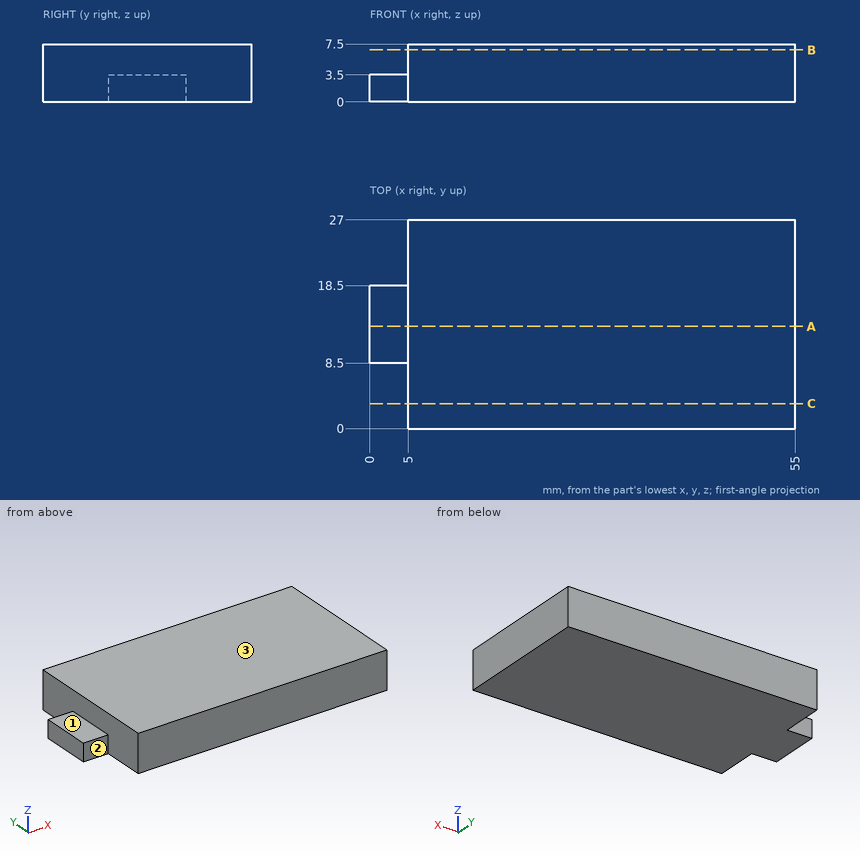
Here's the drawing with two shaded views (mm, measured from the low corner). I have some questions. A direction names the side the tool comes from. Coordinates: 2 decimals unless noted, no trailing zeros. Loops run counter-clockwise (first coordinate to the right, second up) from the corner with the lowest first, then second, coordinate; pieces in that order, holes last. Notation, with made-up numbers: (34, -6.5) -> (61, -6.5) arc R32 ccw to (61, 21.5) -> close; hole circle Ø3 at (-33.75, 30.25). An arc over 180 degrees is marked (long way). Put each result on its own line as item: value. Start each with the question number.
Q1. If I drill on line 1 (X direction, y = 12.25, z = 5.75), over which ranges is the centre line in solid material (lowest first)? Write a range as [from, to].
Q2. I want a section at C-C (y = 3.25). Write out the boundary of the cut face in (x, z).
Q3. I'm going to push flat-ended pins straight in: P1, Ø1.5, axis at x = 13.5, z = 5, coming from the -Y side; P2, Ø1.8, axis at x = 3, z = 2, coming from the +Y side; P3, Ø1.5, axis at y = 23.5, z = 5.5, coming from the -X side; P4, Ø1.5, axis at x = 3.5, y = 14.5, coming from the +Z side. Where does each tip first touch, or does it pass through?
Q4. I want a section at B-B (z = 6.75). Write out the boundary of the cut face in (x, y).
Q5. I want a section at A-A (y = 13.25). Write out the boundary of the cut face in (x, z).
Q6. For the marked faces 1, 2 and 3, which set-ups out of +Z, -Z, +X, -X, +Y, -Y let a thin tool reach every point of the face, with its end or its side?
Taken from the geometry:
1. line 1: x = [5, 55]
2. outline: (5, 0) -> (55, 0) -> (55, 7.5) -> (5, 7.5) -> close
3. P1: stops at y = 0
3. P2: stops at y = 18.5
3. P3: stops at x = 5
3. P4: stops at z = 3.5
4. outline: (5, 0) -> (55, 0) -> (55, 27) -> (5, 27) -> close
5. outline: (0, 0) -> (55, 0) -> (55, 7.5) -> (5, 7.5) -> (5, 3.5) -> (0, 3.5) -> close
6. face 1: +Z, -X, +Y, -Y
6. face 2: +Z, -Z, -X, -Y
6. face 3: +Z, +X, -X, +Y, -Y
